```python
from build123d import *

# Parameters (mm, degrees)
F0_W     = 1044
F0_H     = 389
F1_DEPTH = 288
F3_DEPTH = 389
F4_R     = 100
F5_R     = 15
F6_DEPTH = 50


with BuildPart() as f1:
    # F0 (on Top) → F1 (new body)
    with BuildSketch(Plane.XY):
        Rectangle(F0_W, F0_H)
    extrude(amount=F1_DEPTH)

    # F2 (on face) → F3 (cut, through all)
    with BuildSketch(Plane.XZ.offset(194.5)):
        Polygon((522, 288), (329.74236, 288), (522, 177), align=None)
    extrude(amount=-F3_DEPTH, mode=Mode.SUBTRACT)

    # F4
    f4_edges = [f1.edges().sort_by_distance(p)[0] for p in [
        (-522, 194.5, 144),
        (-522, -194.5, 144),
        (-522, 0, 0),
        (-522, 0, 288),
    ]]
    fillet(f4_edges, radius=F4_R)

    # F5 (on face) → F6 (join)
    with BuildSketch(Plane(origin=(0, 0, 0), x_dir=(1, 0, 0), z_dir=(0, 0, -1))):
        with Locations((150, 163.5)):
            Circle(F5_R)
        with Locations((-321, 163.5)):
            Circle(F5_R)
        with Locations((-321, -163.5)):
            Circle(F5_R)
        with Locations((150, -163.5)):
            Circle(F5_R)
    extrude(amount=F6_DEPTH)


with BuildPart() as f1_1:
    # F7: moved
    add(f1.part.moved(Location((0, 0, 50))))


solid = f1_1.part
```
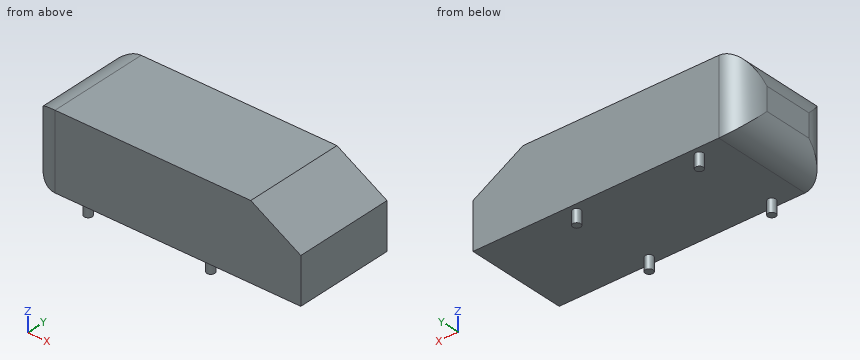
Source: CAD feature listing. Evaluate the final solid. Frame: model axes, mm. Round coordinates to 2 decimals unless told otherwise and drop trailing zeros. Loops run counter-clockwise (first coordinate to the right, second up) from the corner with the lowest first, then second, coordinate; pieces in that order, holes last.
(1) Material intervals for probe 1 along X at (y, z) = (-165, 15.5); probe 2 along Z at (x, y) = (200, 127); probe 3 along X at (y, z) = (74, 233), sorted ascending.
From the geometry:
probe 1: x = -335.92 to -306.08, 135.08 to 164.92
probe 2: z = 50 to 338
probe 3: x = -522 to 511.61
(2) Section query B-B (z = 37). Output: boundary loops of the cut face in (x, y), and give its area (3 significant figures).
From the geometry:
outline: circle Ø30 at (-321, -163.5); circle Ø30 at (-321, 163.5); circle Ø30 at (150, -163.5); circle Ø30 at (150, 163.5)
area: 2,830 mm2
(3) Section query C-C (y = 163.5). Output: boundary loops of the cut face in (x, z), and give its area (3 significant figures).
From the geometry:
outline: (-494.38, 81) arc R100 ccw to (-422, 50) - (-336, 50) - (-336, 0) - (-306, 0) - (-306, 50) - (135, 50) - (135, 0) - (165, 0) - (165, 50) - (522, 50) - (522, 227) - (329.74, 338) - (-422, 338) arc R100 ccw to (-494.38, 307) - close
area: 284,000 mm2
(4) Section query A-A (x = -321). Output: boundary loops of the cut face in (y, z).
From the geometry:
outline: (-194.5, 50) - (-178.5, 50) - (-178.5, 0) - (-148.5, 0) - (-148.5, 50) - (148.5, 50) - (148.5, 0) - (178.5, 0) - (178.5, 50) - (194.5, 50) - (194.5, 338) - (-194.5, 338) - close
(5) Section query D-D (z = 261.5). Output: boundary loops of the cut face in (x, y).
From the geometry:
outline: (-519.2, -118) arc R100 ccw to (-422, -194.5) - (462.24, -194.5) - (462.24, 194.5) - (-422, 194.5) arc R100 ccw to (-519.2, 118) - close
(6) Contact query for flat-ended pins moving along their axis: pin 1 Ø10 at (y, z) = (147.5, 41) entering from -X; pin 2 Ø4 at (y, z) = (16, 102.5) entering from -X. Output: stop coordinate, or through.
From the geometry:
pin 1: stops at x = -331.2
pin 2: stops at x = -511.05
